from build123d import *

# Parameters (mm, degrees)
F0_W     = 127
F0_H     = 127
F0_W_2   = 20.828
F0_H_2   = 1.778
F0_W_3   = 1.778
F0_H_3   = 20.828
F1_DEPTH = 3.175


with BuildPart() as f1:
    # F0 (on Top) → F1 (new body)
    with BuildSketch(Plane.XY):
        Rectangle(F0_W, F0_H)
        with Locations((-25.4, -51.435)):
            Rectangle(F0_W_2, F0_H_2, mode=Mode.SUBTRACT)
        with Locations((-51.435, -25.4)):
            Rectangle(F0_W_3, F0_H_3, mode=Mode.SUBTRACT)
        with Locations((25.4, -51.435)):
            Rectangle(F0_W_2, F0_H_2, mode=Mode.SUBTRACT)
        with Locations((51.435, -25.4)):
            Rectangle(F0_W_3, F0_H_3, mode=Mode.SUBTRACT)
        with Locations((-51.435, 25.4)):
            Rectangle(F0_W_3, F0_H_3, mode=Mode.SUBTRACT)
        with Locations((-25.4, 51.435)):
            Rectangle(F0_W_2, F0_H_2, mode=Mode.SUBTRACT)
        with Locations((51.435, 25.4)):
            Rectangle(F0_W_3, F0_H_3, mode=Mode.SUBTRACT)
        with Locations((25.4, 51.435)):
            Rectangle(F0_W_2, F0_H_2, mode=Mode.SUBTRACT)
    extrude(amount=F1_DEPTH)


solid = f1.part
CAD build for the part. Positions are in the model's coordinates, mm. A direction names the side the tool comes from. Coordinates: 2 decimals unless noted, no trailing zeros. Order: outer loops, then holes, each group sorted by start corner. A loop starts at its lowest first (then second) coordinate and runs counter-clockwise, first axis right, second up.
Item 1: Drill centre line: L1, parallel to X at y = -31.5, z = 0.8. Where is it in solid material? Low to high.
Check sheet entries:
L1: x = -63.5 to -52.32, -50.55 to 50.55, 52.32 to 63.5
Item 2: 3-axis set-ups, long thin cutter, end or side, ignore diameter. For faces 5 (the face through (-1, -63.5, 2)), 6 (the face through (-26, -50.546, 2)): which of +Z, -Z, +X, -X, +Y, -Y reach the whole face in a straight line?
Check sheet entries:
face 5: +Z, -Z, +X, -X, -Y
face 6: +Z, -Z
Item 3: Two-plate mould, pull along X, no slides. Class faces 1 (the face through (-26, 50.546, 2)), 2 (the face through (25, -52.324, 2)), 3 (the face through (-63.5, -1, 2)), 4 (the face through (63.5, -1, 2)): +X half, -X half, draft (parallel to the pull), parting line (faces both ways), or undercut.
Check sheet entries:
face 1: undercut
face 2: undercut
face 3: -X half
face 4: +X half
Item 4: Band-saw the part on C-C on z = 1.75. Give the number of separate pieces and of enclosed holes in the cut face, plus the area to 3 significant figures.
Check sheet entries:
separate pieces: 1
enclosed holes: 8
area: 15,800 mm2
Item 5: Band-saw the part on A-A on x = 24.5. List the corners of the cut face in (y, z) (3 decimals).
Check sheet entries:
outline: (-63.5, 0) - (-52.324, 0) - (-52.324, 3.175) - (-63.5, 3.175) - close; (-50.546, 0) - (50.546, 0) - (50.546, 3.175) - (-50.546, 3.175) - close; (52.324, 0) - (63.5, 0) - (63.5, 3.175) - (52.324, 3.175) - close
